Geometry check sheet. Reference: drawing and pictorial views, mm from the part's lowest x, y, z. A direction names the side the tool comes from. Coordinates: 2 decimals unless noted, no trailing zeros. Loops run counter-clockwise (first coordinate to the right, second up) from the corner with the lowest first, then second, coordinate; pieces in that order, holes last.
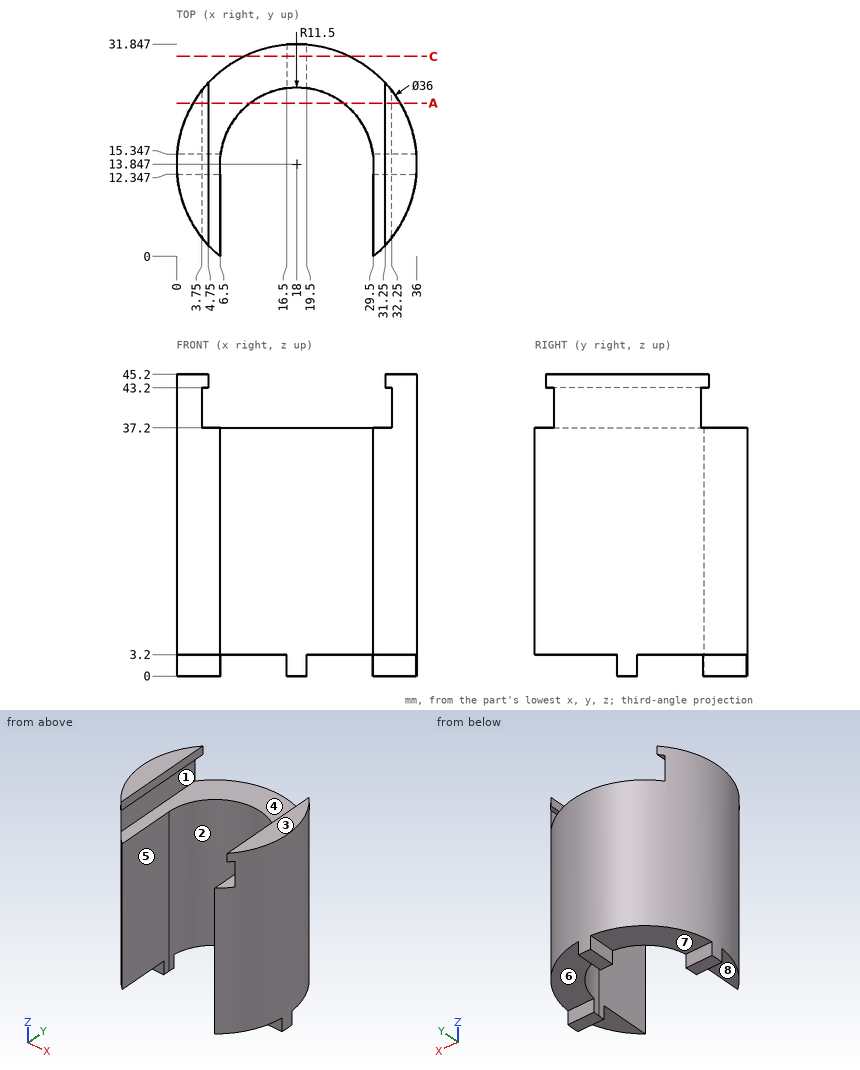
1) Material ranges on probe 1 along X at (y, z) = (14, 30.5); probe 2 along Y at (x, z) = (18, 33.5); probe 3 along Z at (x, y) = (30, 20.5), recorded low to high.
Data:
probe 1: x = 0 to 6.5, 29.5 to 36
probe 2: y = 25.35 to 31.85
probe 3: z = 3.2 to 37.2
2) Access from +Z, -Z, +X, -X, +Y, -Y to the whole of each face (thin tool, end or side, straight path). Record for the marked faces 5, 6, 7 and 8.
Data:
face 5: +Z, -Z, -Y
face 6: -Z, +X, +Y
face 7: -Z, -X, +Y
face 8: -Z, +X, -X, -Y
3) Depth check by flat-ended pin: pin 1 (8 mm diameter, centred on y = 19, z = 22.5, fed in from +X); pin 2 (14.5 mm diameter, centred on x = 22, y = 21, fed in from +Z); pin 3 (12 mm diameter, centred on y = 23, z = 9, fed in from -X). Enter the tip coordinate at first touch or a pass-through.
Data:
pin 1: stops at x = 35.96
pin 2: stops at z = 37.2
pin 3: stops at x = 0.28
4) Section check C-C on y = 30. Record the cut outline in (x, z), and give its area (3 significant figures).
Data:
outline: (10.06, 3.2) - (16.5, 3.2) - (16.5, 0) - (19.5, 0) - (19.5, 3.2) - (25.94, 3.2) - (25.94, 37.2) - (10.06, 37.2) - close
area: 550 mm2
5) Section check A-A on y = 23. Record the cut outline in (x, z).
Data:
outline: (2.5, 3.2) - (11.04, 3.2) - (11.04, 37.2) - (3.75, 37.2) - (3.75, 43.2) - (4.75, 43.2) - (4.75, 45.2) - (2.5, 45.2) - close; (24.96, 3.2) - (33.5, 3.2) - (33.5, 45.2) - (31.25, 45.2) - (31.25, 43.2) - (32.25, 43.2) - (32.25, 37.2) - (24.96, 37.2) - close
6) Mould release check, pull along Z, two halves, no side actions. Record for the marked faces 1, 2, 3 and 4: +Z half, -Z half, draft (parallel to the pull), parting line (faces both ways), or undercut.
Data:
face 1: undercut
face 2: draft
face 3: +Z half
face 4: undercut
